Geometry check sheet. Reference: the model listing, model coordinates, mm. Face numbers are marked on the shaded views. A direction names the side the tool comes from. Round coordinates to 2 decimals unless told otherwise and drop trailing zeros. Order: outer loops, then holes, each group sorted by start corner. A loop starts at its lowest first (then second) coordinate and runs counter-clockwise, first axis right, second up. Notation, with made-up numbers: (-24.5, -34) - (-17.5, -34) arc R21 ccw to (-17.5, -12) - close; hole circle Ø8 at (26, 64). An arc over 180 degrees is marked (long way). One line per question, with ' | ' between items. Start each with the question number.
Q1. Sectioned sample at C-C, the plane x = 123.5. Enter the section's corners in (y, z).
Q2. Sectioned sample at B-B, the plane z = -4. Enter the section's corners in (x, y), then the cut area to 3 significant figures.
Q3. Material ranges on line 1 along X through (y, z) = (40.5, 0.25); line 2 along Z through (x, y) = (110, 62); line 3 along X through (y, z) = (23.5, -0.5), recorded low to high.
Q4. Tool access check on the marked faces 1 and 2. Record the directions out of +Z, -Z, +X, -X, +Y, -Y that give a thin tool (end or side, any length) a straight path to the whole face; none if there is none.
Q5. Gauge pin test, flat ends, axial feed: P1, Ø11, axis at x = 14.47, y = -14.29, coming from the -Z side; P2, Ø2.5, axis at y = 11.06, z = -4, coming from the -X side; P3, Ø6, axis at x = 141.07, y = -14.29, coming from the -Z side; P4, Ø6.5, axis at y = 10.5, z = -4, coming from the +X side. Record the tip position at first contact, or that the pin passes through.
Q6. Sectioned sample at A-A, the plane x = 83. Enter the section's corners in (y, z).
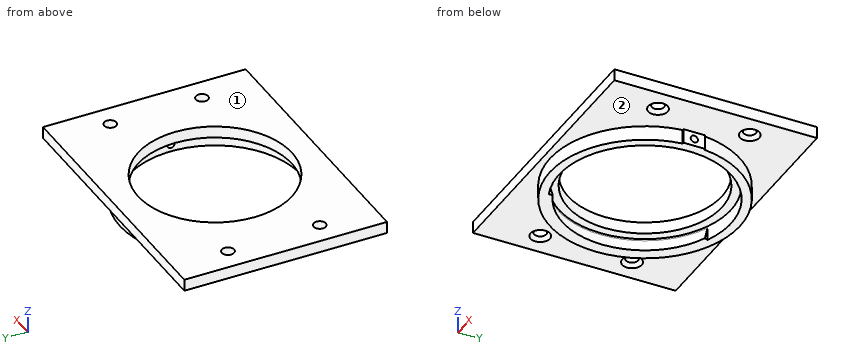
Autodesk Inventor part; units mm, degrees
ref_plane "YZ Plane" through (0, 0, 0) normal (1, 0, 0) x (0, 1, 0)
ref_plane "XZ Plane" through (0, 0, 0) normal (0, 1, 0) x (-1, 0, 0)
ref_plane "XY Plane" through (0, 0, 0) normal (0, 0, 1) x (1, 0, 0)
sketch "Sketch1" plane through (0, 0, 0) normal (0, 0, 1) x (1, 0, 0)
  line L0 (14.4686, 36.4073) -> (141.0686, 36.4073) construction
  line L1 (141.0686, 36.4073) -> (141.0686, -14.2927) construction
  line L2 (141.0686, -14.2927) -> (14.4686, -14.2927) construction
  line L3 (14.4686, -14.2927) -> (14.4686, 36.4073) construction
  circle A0 centre (14.4686, 36.4073) radius 3.375
  circle A1 centre (14.4686, -14.2927) radius 3.375
  circle A2 centre (141.0686, -14.2927) radius 3.375
  circle A3 centre (141.0686, 36.4073) radius 3.375
  line L4 (1.7686, 67.0573) -> (153.7686, 67.0573)
  line L5 (153.7686, 67.0573) -> (153.7686, -44.9427)
  line L6 (153.7686, -44.9427) -> (1.7686, -44.9427)
  line L7 (1.7686, -44.9427) -> (1.7686, 67.0573)
  line L8 (14.4686, 36.4073) -> (1.7686, 67.0573) construction
  line L9 (14.4686, -14.2927) -> (1.7686, -44.9427) construction
  line L10 (141.0686, -14.2927) -> (153.7686, -44.9427) construction
  line L11 (141.0686, 36.4073) -> (153.7686, 67.0573) construction
  line L12 (153.7686, 11.0573) -> (1.7686, 11.0573) construction
  point P0 (0, 0)
  dimension "d1" = 126.6
  dimension "d2" = 50.7
  dimension "d3" = 6.75
  dimension "d4" = 152
  dimension "d5" = 112
extrude "Extrusion1" add sketch "Sketch1" along normal blind 6.5
sketch "Sketch4" plane through (0, 0, 0) normal (0, 0, -1) x (-1, 0, 0)
  circle A0 centre (-77.7686, 11.0573) radius 47.5
  line L0 (-153.7686, 67.0573) -> (-1.7686, 67.0573) construction
  line L1 (-1.7686, -44.9427) -> (-153.7686, -44.9427) construction
  line L2 (-1.7686, 67.0573) -> (-153.7686, -44.9427) construction
  line L3 (-1.7686, -44.9427) -> (-153.7686, 67.0573) construction
  circle A1 centre (-77.7686, 11.0573) radius 52.5
  circle A2 centre (-77.7686, 11.0573) radius 42.5
  point P0 (0, 0)
  dimension "d12" = 95
  dimension "d13" = 5
  dimension "d34" = 5
extrude "Extrusion2" add sketch "Sketch4" along normal blind 8 contours A1
ref_plane "Work Plane3" through (1.7686, 11.0573, 0) normal (0, -1, 0) x (1, 0, 0)
sketch "Sketch6" plane through (1.7686, 11.0573, 0) normal (0, -1, 0) x (1, 0, 0)
  line L0 (28.5, 0) -> (28.5, -8)
  line L1 (123.5, -8) -> (28.5, -8)
  line L2 (28.5, -8) -> (30.5, -8)
  line L3 (30.5, -8) -> (28.5, -1)
  line L4 (28.5, -8) -> (28.5, -1)
  line L5 (76, -10.9) -> (76, 9.4)
  dimension "d16" = 2
  dimension "d17" = 7
revolve "Revolution1" add sketch "Sketch6" angle 135 mid plane about axis through (77.7686, 11.0573, -8) along (0, 0, 1)
ref_plane "Work Plane4" through (130.2686, 11.0573, 0) normal (1, 0, 0) x (0, 1, 0)
sketch "Sketch7" plane through (130.2686, 11.0573, 0) normal (1, 0, 0) x (0, 1, 0)
  line L0 (-52.5, -8) -> (52.5, -8)
  line L1 (56, 0) -> (-56, 0)
  line L2 (56, 0) -> (56, 6.5)
  line L3 (-56, 6.5) -> (56, 6.5)
  line L4 (-56, 0) -> (-56, 6.5)
  line L5 (47.5, -8) -> (-47.5, -8)
  line L6 (-47.5, 0) -> (47.5, 0)
  line L7 (6, -8) -> (-6, -8)
  line L8 (-6, -8) -> (-6, 0)
  line L9 (-6, 0) -> (6, 0)
  line L10 (6, 0) -> (6, -8)
  line L11 (0, -10.9) -> (0, 9.4)
  circle A0 centre (0, -4) radius 2
  point P0 (-11.0573, 0)
  point P1 (-43.8843, -8)
  point P2 (43.8843, -8)
  point P3 (0, -8)
  dimension "d23" = 12
  dimension "d24" = 4
extrude "Extrusion3" add sketch "Sketch7" against normal up to next contours L8 L1 L11 A0 L0 | L11 A0 L1 L10 L0
extrude "Extrusion4" add sketch "Sketch7" along normal blind 0.5 contours L8 L1 L11 A0 L0 | L11 A0 L1 L10 L0
extrude "Extrusion5" cut sketch "Sketch7" against normal up to next contours A0 L11 | L11 A0
chamfer "Chamfer1" distance 2 angle 45 4 edges at (11.0936, -14.2927, 0) (11.0936, 36.4073, 0) (137.6936, 36.4073, 0) (137.6936, -14.2927, 0)
extrude "Extrusion6" cut sketch "Sketch4" against normal through all contours A2
properties part number "AZ100 ASI LX-4000 stage adapter"
Determined:
1) outline: (-44.94, 0) - (-14.73, 0) - (-14.73, -8) - (-1.78, -8) - (-1.78, 0) - (23.9, 0) - (23.9, -8) - (36.84, -8) - (36.84, 0) - (67.06, 0) - (67.06, 6.5) - (-44.94, 6.5) - close
2) outline: (59.59, -32.83) - (59.92, -32.04) arc R46.64 cw to (59.92, 54.15) - (59.59, 54.94) arc R47.5 cw to (125.23, 13.06) - (130.77, 13.06) - (130.77, 17.06) - (129.92, 17.06) arc R52.5 ccw (long way) to (129.92, 5.06) - (130.77, 5.06) - (130.77, 9.06) - (125.23, 9.06) arc R47.5 cw to start | area: 1,650 mm2
3) line 1: x = 1.77 to 11.38, 17.55 to 47.12, 108.42 to 137.98, 144.15 to 153.77 | line 2: z = 0 to 6.5 | line 3: x = 26.76 to 31.93, 123.61 to 128.77
4) face 1: +Z, +X, -X, +Y, -Y | face 2: -Z
5) P1: stops at z = 0 | P2: stops at x = 25.27 | P3: passes through | P4: stops at x = 130.77
6) outline: (-44.94, 0) - (-41.18, 0) - (-41.18, -8) - (-36.15, -8) - (-36.15, 0) - (-31.12, 0) - (-31.12, 6.5) - (-44.94, 6.5) - close; (53.23, 0) - (58.27, 0) - (58.27, -8) - (63.3, -8) - (63.3, 0) - (67.06, 0) - (67.06, 6.5) - (53.23, 6.5) - close
